The model under review builds one solid part; all positions refer to its coordinate system, in mm. Face numbers are marked on the shaded views. Coordinates: 2 decimals unless noted, no trailing zeros. Order: outer loops, then holes, each group sorted by start corner. A loop starts at its lowest first (then second) coordinate and runs counter-clockwise, first axis right, second up. Notation, with made-up numbers: (55, 79) - (76, 79) arc R36 cw to (76, 113) - close; hole circle Ø8 at (7.5, 49.25). An arc over 180 degrees is marked (long way). Answer in a Markdown table with one row per item.
```python
from build123d import *

# Parameters (mm, degrees)
SKETCH_1_W            = 45
SKETCH_1_H            = 24.2
EXTRUDE_1_DEPTH       = 3
FILLET_1_R            = 3
HOLE_WIZARD_M31_D     = 3.4
HOLE_WIZARD_M31_DEPTH = 3
HOLE_WIZARD_M31_TIP   = 1.021463052
CUT_EXTRUDE_1_DEPTH   = 1
FILLET_2_R            = 2
SKETCH_3_W            = 7
SKETCH_3_H            = 7
CUT_EXTRUDE_2_DEPTH   = 2.2
FILLET_3_R            = 2


with BuildPart() as part:
    # Эскиз1 → Бобышка-Вытянуть1 (new body)
    with BuildSketch(Plane(origin=(0, 0, 0), x_dir=(1, 0, 0), z_dir=(0, 1, 0))):
        with Locations((22.5, 12.1)):
            Rectangle(SKETCH_1_W, SKETCH_1_H)
    extrude(amount=EXTRUDE_1_DEPTH)

    # Скругление1
    fillet_1_edges = [part.edges().sort_by_distance(p)[0] for p in [
        (0, 1.5, -24.2),
        (45, 1.5, -24.2),
        (45, 1.5, 0),
        (0, 1.5, 0),
    ]]
    fillet(fillet_1_edges, radius=FILLET_1_R)

    # Отверстие с зазором M31
    with Locations(Plane(origin=(69.423819873, 0, -24.090135757), x_dir=(0, 0, 1), z_dir=(0, -1, 0))):
        with Locations((2.890135757, 66.423819873), (21.090135757, 66.423819873), (11.990135757, 27.423819873)):
            Hole(HOLE_WIZARD_M31_D / 2, depth=HOLE_WIZARD_M31_DEPTH)
            with Locations((0, 0, -(HOLE_WIZARD_M31_DEPTH + HOLE_WIZARD_M31_TIP / 2))):  # 118° drill point
                Cone(0, HOLE_WIZARD_M31_D / 2, HOLE_WIZARD_M31_TIP, mode=Mode.SUBTRACT)

    # Эскиз7 → Вырез-Вытянуть1 (cut)
    with BuildSketch(Plane(origin=(0, 3, 0), x_dir=(1, 0, 0), z_dir=(0, 1, 0))):
        with BuildLine():
            Line((2, 8.123475383), (2, 16.076524617))
            ThreePointArc((2, 16.076524617), (2.522831528, 17.768752841), (3.909090909, 18.871147553))
            ThreePointArc((3.909090909, 18.871147553), (4.767766953, 19.432233047), (5.328852447, 20.290909091))
            ThreePointArc((5.328852447, 20.290909091), (6.431247159, 21.677168472), (8.123475383, 22.2))
            Line((8.123475383, 22.2), (36.752647357, 22.2))
            Line((36.752647357, 22.2), (36.752647357, 2))
            Line((36.752647357, 2), (8.123475383, 2))
            ThreePointArc((8.123475383, 2), (6.431247159, 2.522831528), (5.328852447, 3.909090909))
            ThreePointArc((5.328852447, 3.909090909), (4.767766953, 4.767766953), (3.909090909, 5.328852447))
            ThreePointArc((3.909090909, 5.328852447), (2.522831528, 6.431247159), (2, 8.123475383))
        make_face()
    extrude(amount=-CUT_EXTRUDE_1_DEPTH, mode=Mode.SUBTRACT)

    # Скругление2
    fillet_2_edges = [part.edges().sort_by_distance(p)[0] for p in [
        (36.752647357, 2.5, -22.2),
        (36.752647357, 2.5, -2),
    ]]
    fillet(fillet_2_edges, radius=FILLET_2_R)

    # Эскиз3 → Вырез-Вытянуть2 (cut)
    with BuildSketch(Plane(origin=(0, 3, 0), x_dir=(1, 0, 0), z_dir=(0, 1, 0))):
        with Locations((3.5, 12.1)):
            Rectangle(SKETCH_3_W, SKETCH_3_H)
    extrude(amount=-CUT_EXTRUDE_2_DEPTH, mode=Mode.SUBTRACT)

    # Скругление3
    fillet_3_edges = [part.edges().sort_by_distance(p)[0] for p in [
        (7, 1.4, -8.6),
        (7, 1.4, -15.6),
    ]]
    fillet(fillet_3_edges, radius=FILLET_3_R)


solid = part.part
```
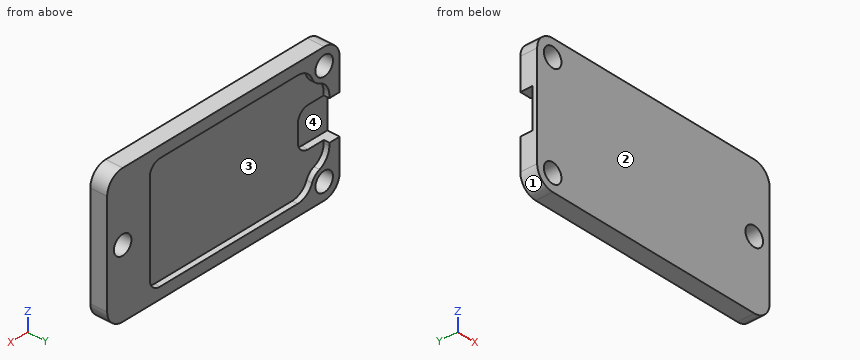
Item 1: Clearance check with flat-ended pins moving along their axes: pin 1 Ø3.5 at (x, z) = (4, -11) entering from +Y; pin 2 Ø4 at (x, z) = (3, -3) entering from -Y; pin 3 Ø1.1 at (x, y) = (1.5, 2) entering from +Z; pin 4 Ø0.7 at (x, y) = (2.5, 2.5) entering from -Z. State where each tip first meets the part, or that it passes through.
Check values:
| item | result |
|---|---|
| pin 1 | y = 0.8 |
| pin 2 | y = 0 |
| pin 3 | z = -0.15 |
| pin 4 | z = -24.2 |
Item 2: To check wall thickness, follow line 1 (X direction, y = 0.8, z = -21.2); line 2 (Z direction, x = 31.5, y = 2.4); line 3 (Z direction, x = 42, y = 1.45). State the ranges of each line that lie inside material, in increasing order. Write a range as from..to.
Check values:
| item | result |
|---|---|
| line 1 | 0..1.3, 4.7..45 |
| line 2 | -24.2..-22.2, -2..0 |
| line 3 | -24.2..-13.8, -10.4..0 |
Item 3: We need section B-B, the plane x = 34. Write out the cut boundary in (y, z).
Check values:
| item | result |
|---|---|
| outline | (0, -24.2) - (3, -24.2) - (3, -22.2) - (2, -22.2) - (2, -2) - (3, -2) - (3, 0) - (0, 0) - close |
Item 4: We need section C-C, the plane z = -15. Write out the cut boundary in (x, y).
Check values:
| item | result |
|---|---|
| outline | (0, 0) - (45, 0) - (45, 3) - (36.75, 3) - (36.75, 2) - (6.43, 2) - (6.43, 0.8) - (0, 0.8) - close |
Item 5: We need section A-A, the plane z = -12.1. Write out the cut boundary in (x, y).
Check values:
| item | result |
|---|---|
| outline | (0, 0) - (40.3, 0) - (40.3, 3) - (36.75, 3) - (36.75, 2) - (7, 2) - (7, 0.8) - (0, 0.8) - close; (43.7, 0) - (45, 0) - (45, 3) - (43.7, 3) - close |
Item 6: Mouldability with a two-part tool opening along Z and no side actions: class the marked faces 1, 2, 3 and 4 as +Z half, -Z half, draft (parallel to the pull), parting line (faces both ways), or undercut.
Check values:
| item | result |
|---|---|
| face 1 | -Z half |
| face 2 | draft |
| face 3 | undercut |
| face 4 | undercut |
